Input: part model. Units: mm. Frame: model coordinates. A direction names the side the tool comes from. Round coordinates to 2 decimals unless told otherwise and drop trailing zeros. Write each loop counter-clockwise with the first axis right and the second up, starting at its lowest first coordinate (ties: lowest second). Pieces come first, ordered by that corner, then holes. Notation, with made-up numbers: (-14.5, -32.75) -> (32.5, -32.75) arc R22 ccw to (32.5, -20.75) -> close; hole circle Ø1 at (89.5, 74). An arc over 180 degrees is marked (long way). Use CSV: the item, a comma, the result in double quotes.
Autodesk Inventor part; units mm, degrees
ref_plane "YZ Plane" through (0, 0, 0) normal (1, 0, 0) x (0, 1, 0)
ref_plane "XZ Plane" through (0, 0, 0) normal (0, 1, 0) x (-1, 0, 0)
ref_plane "XY Plane" through (0, 0, 0) normal (0, 0, 1) x (1, 0, 0)
sketch "Sketch5" plane through (0, 0, 0) normal (0, 0, 1) x (1, 0, 0)
  circle A0 centre (0, 0) radius 11.251
  dimension "d8" = 22.502
extrude "Extrusion5" add sketch "Sketch5" along normal blind 4
sketch "Sketch6" plane through (0, 0, 4) normal (0, 0, 1) x (1, 0, 0)
  circle A0 centre (0, 0) radius 11.251
  circle A1 centre (0, 0) radius 5
  dimension "d15" = 10
extrude "Extrusion6" add sketch "Sketch6" along normal blind 4 contours A1
hole "Hole1" at (0, 0, 0) direction (0, 0, 1) diameter 4.5 end through all
chamfer "Chamfer2" distance 0.5 angle 45 3 edges at (-11.251, 0, 0) (-11.251, 0, 4) (-5, 0, 8)
properties part number "BC-10011" material "Aço Inox AISI 304"
Item 1: First-contact query: pin 1 Ø1 at (x, z) = (4, 1.5) entering from -Y. Flat tip, straight axial feed; report the tip coordinate or a pass-through.
Worked answers:
pin 1,"stops at y = -10.69"
Item 2: Section query D-D on z = 3. Return the cut outline in (x, y), plus the area to 3 significant figures.
Worked answers:
outline,"circle Ø22.5 at (0, 0); hole circle Ø4.5 at (0, 0)"
area,"382 mm²"
Item 3: Set-up query: faces 1 (the face through (-1.08, 4.88, 5.73)), 2 (the face through (0, 3, 0)). Return all of +Z, -Z, +X, -X, +Y, -Y with unobstructed straight access to the full face (end or side cutting, diameter ignored); none if empty.
Worked answers:
face 1,"+Z"
face 2,"-Z, +X, -X, +Y, -Y"
Item 4: Pull-direction query (Y, two-part tool) for faces 3 (the face through (10.73, -3.38, 1.98)), 4 (the face through (-2.23, -0.29, 4.06)), 5 (the face through (5, -2, 4)); classes: +Y half, -Y half, draft (parallel to the pull), parting line (faces both ways), or undercut.
Worked answers:
face 3,"parting line"
face 4,"undercut"
face 5,"draft"
Item 5: Line query: line 1 (Y direction, x = 0, z = 4.75); line 2 (Z direction, x = 3, y = -8.5); line 3 (Y direction, x = 0, z = 2.5). Output: solid intervals per line, ascending.
Worked answers:
line 1,"y = -5 to -2.25, 2.25 to 5"
line 2,"z = 0 to 4"
line 3,"y = -11.25 to -2.25, 2.25 to 11.25"
Item 6: Section query A-A on x = 0. Return the cut outline in (y, z), plus the area to 3 significant figures.
Worked answers:
outline,"(-11.25, 0.5) -> (-10.75, 0) -> (-2.25, 0) -> (-2.25, 8) -> (-4.5, 8) -> (-5, 7.5) -> (-5, 4) -> (-10.75, 4) -> (-11.25, 3.5) -> close; (2.25, 0) -> (10.75, 0) -> (11.25, 0.5) -> (11.25, 3.5) -> (10.75, 4) -> (5, 4) -> (5, 7.5) -> (4.5, 8) -> (2.25, 8) -> close"
area,"93.3 mm²"
Item 7: Section query C-C on z = 4.75. Return the cut outline in (x, y), plus the area to 3 significant figures.
Worked answers:
outline,"circle Ø10 at (0, 0); hole circle Ø4.5 at (0, 0)"
area,"62.6 mm²"
